from build123d import *

# Parameters (mm, degrees)
SKETCH1_W                       = 134.9248
SKETCH1_H                       = 57.15
BOSS_EXTRUDE1_DEPTH             = 4.7625
CUT_EXTRUDE1_DEPTH              = 10.525
F_10_24_TAPPED_HOLE1_AT_2_COUNT = 2
F_10_24_TAPPED_HOLE1_AT_2_PITCH = 44.45
FILLET1_R                       = 1.905


with BuildPart() as part:
    # Sketch1 → Boss-Extrude1 (new body, symmetric)
    with BuildSketch(Plane.XY):
        Rectangle(SKETCH1_W, SKETCH1_H)
    extrude(amount=BOSS_EXTRUDE1_DEPTH, both=True)

    # Sketch3 → Cut-Extrude1 (cut, through all)
    with BuildSketch(Plane.XY.offset(4.7625)):
        with BuildLine():
            Line((-61.1124, 8.609886798), (-61.1124, -8.609886798))
            ThreePointArc((-61.1124, -8.609886798), (-57.664894583, -15.155408542), (-50.317097979, -16.015079156))
            Line((-50.317097979, -16.015079156), (-24.169295524, -5.924153886))
            ThreePointArc((-24.169295524, -5.924153886), (-20.105537141, 0), (-24.169295524, 5.924153886))
            Line((-24.169295524, 5.924153886), (-50.317097979, 16.015079156))
            ThreePointArc((-50.317097979, 16.015079156), (-57.664894583, 15.155408542), (-61.1124, 8.609886798))
        make_face()
        with BuildLine():
            Line((-31.725706947, -22.225), (31.725706947, -22.225))
            ThreePointArc((31.725706947, -22.225), (34.847022318, -19.631390878), (32.868827755, -16.087923057))
            Line((32.868827755, -16.087923057), (6.85872485, -6.050138615))
            ThreePointArc((6.85872485, -6.050138615), (0, -4.772600274), (-6.85872485, -6.050138615))
            Line((-6.85872485, -6.050138615), (-32.868827755, -16.087923057))
            ThreePointArc((-32.868827755, -16.087923057), (-34.847022318, -19.631390878), (-31.725706947, -22.225))
        make_face()
        with BuildLine():
            Line((-31.725706947, 22.225), (31.725706947, 22.225))
            ThreePointArc((31.725706947, 22.225), (34.847022318, 19.631390878), (32.868827755, 16.087923057))
            Line((32.868827755, 16.087923057), (6.85872485, 6.050138615))
            ThreePointArc((6.85872485, 6.050138615), (0, 4.772600274), (-6.85872485, 6.050138615))
            Line((-6.85872485, 6.050138615), (-32.868827755, 16.087923057))
            ThreePointArc((-32.868827755, 16.087923057), (-34.847022318, 19.631390878), (-31.725706947, 22.225))
        make_face()
        with BuildLine():
            Line((61.1124, 8.609886798), (61.1124, -8.609886798))
            ThreePointArc((61.1124, -8.609886798), (57.664894583, -15.155408542), (50.317097979, -16.015079156))
            Line((50.317097979, -16.015079156), (24.169295524, -5.924153886))
            ThreePointArc((24.169295524, -5.924153886), (20.105537141, 0), (24.169295524, 5.924153886))
            Line((24.169295524, 5.924153886), (50.317097979, 16.015079156))
            ThreePointArc((50.317097979, 16.015079156), (57.664894583, 15.155408542), (61.1124, 8.609886798))
        make_face()
    extrude(amount=-CUT_EXTRUDE1_DEPTH, mode=Mode.SUBTRACT)

    # Sketch4 → #10-24 Tapped Hole1 (revolve, cut)
    with BuildSketch(Plane(origin=(-67.4624, 22.225, 0), x_dir=(0, 0, 1), z_dir=(0, 1, 0))):
        Polygon((0, 0), (0, 14.094824014), (1.89865, 12.954), (1.89865, 0), align=None)
    f_10_24_tapped_hole1 = revolve(axis=Axis((-73.8124, 22.225, 0), (1, 0, 0)), mode=Mode.SUBTRACT)

    # #10-24 Tapped Hole1 at 2: #10-24 Tapped Hole1 ×2
    with Locations(*[(0, -i * F_10_24_TAPPED_HOLE1_AT_2_PITCH, 0) for i in range(1, F_10_24_TAPPED_HOLE1_AT_2_COUNT)]):
        add(f_10_24_tapped_hole1, mode=Mode.SUBTRACT)

    # Mirror1: #10-24 Tapped Hole1 across plane
    add(f_10_24_tapped_hole1.mirror(Plane(origin=(0, 0, 0), x_dir=(0, 0, 1), z_dir=(1, 0, 0))), mode=Mode.SUBTRACT)

    # Mirror1 copy 1 sketch → Mirror1 copy 1 (revolve, cut)
    with BuildSketch(Plane(origin=(67.4624, -22.225, 0), x_dir=(0, 0, 1), z_dir=(0, 1, 0))):
        Polygon((0, 0), (0, -14.094824014), (1.89865, -12.954), (1.89865, 0), align=None)
    revolve(axis=Axis((73.8124, -22.225, 0), (1, 0, 0)), mode=Mode.SUBTRACT)

    # Fillet1
    fillet1_edges = [part.edges().sort_by_distance(p)[0] for p in [
        (67.4624, -28.575, 0),
        (-67.4624, -28.575, 0),
        (-67.4624, 28.575, 0),
        (67.4624, 28.575, 0),
    ]]
    fillet(fillet1_edges, radius=FILLET1_R)


solid = part.part
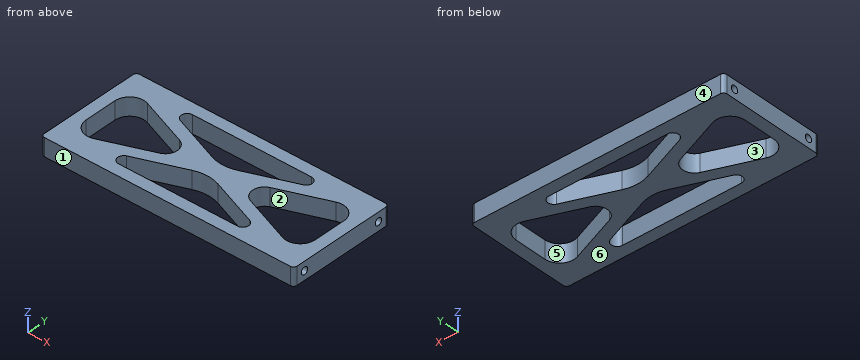
Read the model definition and answer for the solid it produces. Units are mm, in the model's axes. Face numbers are marked on the shaded views. A direction names the side the tool comes from. Give positions to 0.01 mm unless a question says otherwise; leave off trailing zeros. Write each loop counter-clockwise with the first axis right and the second up, starting at its lowest first coordinate (ties: lowest second). Pieces come first, ordered by that corner, then holes. Notation, with made-up numbers: (-6, 44.25) - (32, 44.25) arc R30 cw to (32, 70.25) - close; hole circle Ø9 at (-13.75, 44.5). An arc over 180 degrees is marked (long way). Return JSON: item names as keys, results as strings.
Q1. Consider line 1 along Y through (x, z) = (63.5, 0) (3 decimals); line 2 along X through (y, z) = (2, 2); line 3 along Y through (x, z) = (27.5, -1.75) (3 decimals). Determine where each line is inside the solid, lowest interval first. Write a range as [from, to].
Reply:
{"line 1": "[-28.575, -24.124], [-20.326, 20.326], [24.124, 28.575]", "line 2": "[-67.46, -61.11], [-20.43, 20.43], [61.11, 67.46]", "line 3": "[-28.575, -22.225], [-14.016, -7.21], [7.21, 14.016], [22.225, 28.575]"}
Q2. A cutting plane is placed at A-A, the plane z = -3.5. Count the separate pieces of the cut face and the enclosed holes in it, and give its area (3 significant figures).
Reply:
{"separate pieces": "1", "enclosed holes": "4", "area": "4,170 mm²"}
Q3. Given P1, Ø2.5, axis at y = -22.225, z = 0, coming from the -X side; P2, Ø3, axis at y = -22.225, z = 0, coming from the +X side, each flat-ended and moving along its own axis, determine where each tip first touches the part or whether it passes through.
Reply:
{"P1": "x = -54.12", "P2": "x = 54.27"}
Q4. For the marked faces 5 and 6, determine the directions among +Z, -Z, +X, -X, +Y, -Y from which every point of the face is accessible in a straight line to the end or side of a thin tool.
Reply:
{"face 5": "+Z, -Z", "face 6": "-Z, +X, -X, +Y, -Y"}
Q5. A cutting plane is placed at B-B, the plane x = -57.5. Determine the outline of the cut face in (y, z) (1 decimal), and give its area (3 significant figures).
Reply:
{"outline": "(-28.6, -4.8) - (-15.3, -4.8) - (-15.3, 4.8) - (-28.6, 4.8) - close; (15.3, -4.8) - (28.6, -4.8) - (28.6, 4.8) - (15.3, 4.8) - close; hole circle Ø3.8 at (-22.2, 0); hole circle Ø3.8 at (22.2, 0)", "area": "231 mm²"}
Q6. For a pull along Y with two mould halves and no side action, classify the marked faces 1, 2, 3 and 4 as released by +Y, released by -Y, zero draft, split by the parting line, or undercut.
Reply:
{"face 1": "released by -Y", "face 2": "undercut", "face 3": "undercut", "face 4": "released by +Y"}
Q7. A cutting plane is placed at C-C, the plane x = -22.5. Determine the outline of the cut face in (y, z) (1 decimal).
Reply:
{"outline": "(-28.6, -4.8) - (-22.2, -4.8) - (-22.2, 4.8) - (-28.6, 4.8) - close; (-12.1, -4.8) - (-5, -4.8) - (-5, 4.8) - (-12.1, 4.8) - close; (5, -4.8) - (12.1, -4.8) - (12.1, 4.8) - (5, 4.8) - close; (22.2, -4.8) - (28.6, -4.8) - (28.6, 4.8) - (22.2, 4.8) - close"}
